from build123d import *

# Parameters (mm, degrees)
SKETCH001_W     = 78
SKETCH001_H     = 43
PAD009_DEPTH    = 40
THICKNESS_T     = -3
SKETCH008_W     = 24
SKETCH008_H     = 23
POCKET_DEPTH    = 40.001
CHAMFER009_SIZE = 2
CHAMFER010_SIZE = 0.6


with BuildPart() as part:
    # Sketch001 → Pad009 (new body)
    with BuildSketch(Plane.XY):
        Rectangle(SKETCH001_W, SKETCH001_H)
    extrude(amount=PAD009_DEPTH)

    # Thickness
    thickness_openings = [part.faces().sort_by_distance(p)[0] for p in [
        (0, 0, 0),
    ]]
    offset(amount=THICKNESS_T, openings=thickness_openings)

    # Sketch008 → Pocket (cut, through all)
    with BuildSketch(Plane.XY):
        with Locations((-17, 0)):
            Rectangle(SKETCH008_W, SKETCH008_H)
        with Locations((17, 0)):
            Rectangle(SKETCH008_W, SKETCH008_H)
    extrude(amount=POCKET_DEPTH, mode=Mode.SUBTRACT)

    # Chamfer009
    chamfer009_edges = [part.edges().sort_by_distance(p)[0] for p in [
        (-5, 0, 37),
        (-17, -11.5, 37),
        (-29, 0, 37),
        (17, -11.5, 37),
        (5, 0, 37),
        (29, 0, 37),
        (-17, 11.5, 37),
        (17, 11.5, 37),
    ]]
    chamfer(chamfer009_edges, length=CHAMFER009_SIZE)

    # Chamfer010
    chamfer010_edges = [part.edges().sort_by_distance(p)[0] for p in [
        (-39, 0, 0),
        (0, -21.5, 0),
        (39, 0, 0),
        (0, 21.5, 0),
        (-36, 0, 0),
        (0, 18.5, 0),
        (36, 0, 0),
        (0, -18.5, 0),
        (-39, 0, 40),
        (0, 21.5, 40),
        (0, -21.5, 40),
        (39, 0, 40),
        (17, -11.5, 40),
        (29, 0, 40),
        (17, 11.5, 40),
        (5, 0, 40),
        (-17, -11.5, 40),
        (-5, 0, 40),
        (-17, 11.5, 40),
        (-29, 0, 40),
        (39, 21.5, 20),
        (-39, 21.5, 20),
        (-39, -21.5, 20),
        (39, -21.5, 20),
    ]]
    chamfer(chamfer010_edges, length=CHAMFER010_SIZE)


solid = part.part
Read the model definition and answer for the solid it produces. Units are mm, in the model's axes. A direction names the side the tool comes from. Round coordinates to 2 decimals unless told otherwise and drop trailing zeros. Write each loop counter-clockwise with the first axis right and the second up, starting at its lowest first coordinate (ties: lowest second). Pieces come first, ordered by that corner, then holes.
1. Straight lines are drawn through the part: L1, parallel to X at y = 2.5, z = 23.5; L2, parallel to Y at x = 17, z = 19; L3, parallel to Z at x = 12, y = -15.5. For each, find the intervals that lie inside material, in ascending order.
2. The part is cut by section C-C, the plane z = 27. Determine the outline of the cut face in (x, y).
3. The part is cut by section D-D, the plane y = -16.5. Determine the outline of the cut face in (x, z).
4. Given pin 1 Ø11 at (x, y) = (-15.5, -6.5) entering from -Z; pin 2 Ø5 at (x, y) = (-25, -1) entering from +Z, each flat-ended and moving along its own axis, determine where each tip first touches the part or whether it passes through.
5. Determine the mould class of faces 1 (the face through (39, 0, 20)), 2 (the face through (4, 0, 38)), 3 (the face through (36, 0, 19)), 4 (the face through (-1, 21.5, 20)) for opening direction X: pulls with the +X half, pulls with the -X half, needs draft (parallel to the pull), parting line crosses it, or undercut.
6. The part is cut by section B-B, the plane x = 27. Determine the outline of the cut face in (y, z), then the cut area to 3 significant figures.
7. Which of the six approach directions +Z, -Z, +X, -X, +Y, -Y give full straight-line access (tool end or side, diameter ignored) to faces 5 (the face through (-3, -20, 0)), 6 (the face through (-1, 0, 37))?
8. The part is cut by section A-A, the plane y = -6. State how many separate pieces and enclosed holes the cut face has, then the cut area to 3 significant figures.
Values:
1. L1: x = -39 to -36, 36 to 39
1. L2: y = -21.5 to -18.5, 18.5 to 21.5
1. L3: z = 37 to 40
2. outline: (-39, -20.9) - (-38.4, -21.5) - (38.4, -21.5) - (39, -20.9) - (39, 20.9) - (38.4, 21.5) - (-38.4, 21.5) - (-39, 20.9) - close; hole (-36, -18.5) - (36, -18.5) - (36, 18.5) - (-36, 18.5) - close
3. outline: (-39, 0.6) - (-38.4, 0) - (-36.6, 0) - (-36, 0.6) - (-36, 37) - (36, 37) - (36, 0.6) - (36.6, 0) - (38.4, 0) - (39, 0.6) - (39, 39.4) - (38.4, 40) - (-38.4, 40) - (-39, 39.4) - close
4. pin 1: stops at z = 38.5
4. pin 2: passes through
5. face 1: pulls with the +X half
5. face 2: undercut
5. face 3: undercut
5. face 4: needs draft
6. outline: (-21.5, 0.6) - (-20.9, 0) - (-19.1, 0) - (-18.5, 0.6) - (-18.5, 37) - (-13.5, 37) - (-11.5, 39) - (-11.5, 39.4) - (-12.1, 40) - (-20.9, 40) - (-21.5, 39.4) - close; (11.5, 39) - (13.5, 37) - (18.5, 37) - (18.5, 0.6) - (19.1, 0) - (20.9, 0) - (21.5, 0.6) - (21.5, 39.4) - (20.9, 40) - (12.1, 40) - (11.5, 39.4) - close
6. area: 277 mm2
7. face 5: -Z, +X, -X, +Y, -Y
7. face 6: -Z
8. separate pieces: 3
8. enclosed holes: 0
8. area: 302 mm2
